Model file for the job. Use its own axes, mm. A direction names the side the tool comes from. Coordinates: 2 decimals unless noted, no trailing zeros. Loops run counter-clockwise (first coordinate to the right, second up) from the corner with the lowest first, then second, coordinate; pieces in that order, holes last. Notation, with made-up numbers: (38, 13) -> (92, 13) arc R16 ccw to (92, 29) -> close; hole circle Ø3 at (27, 34.5). An arc over 180 degrees is marked (long way). Use one line per item in the form item = value.
```python
from build123d import *

# Parameters (mm, degrees)
F0_W     = 38
F0_H     = 38
F1_DEPTH = 1.5
F2_R     = 2.25
F2_W     = 2.816632
F2_H     = 26.474444
F2_W_2   = 3.106516
F2_H_2   = 26.623748
F2_W_3   = 2.935091
F2_H_3   = 26.58009
F2_W_4   = 2.913202
F2_H_4   = 26.536286
F3_DEPTH = 1.501
F4_R     = 3
F5_R     = 1


with BuildPart() as f1:
    # F0 (on Top) → F1 (new body)
    with BuildSketch(Plane.XY):
        with Locations((-24.108174, 19)):
            Rectangle(F0_W, F0_H)
    extrude(amount=F1_DEPTH)

    # F2 (on face) → F3 (cut, through all)
    with BuildSketch(Plane.XY.offset(1.5)):
        with Locations((-39.408174, 34.3)):
            Circle(F2_R)
        with Locations((-8.808174, 34.3)):
            Circle(F2_R)
        with Locations((-8.808174, 3.7)):
            Circle(F2_R)
        with Locations((-39.408174, 3.7)):
            Circle(F2_R)
        with Locations((-34.555089, 19.259251)):
            Rectangle(F2_W, F2_H)
        with Locations((-27.583793, 19.268872)):
            Rectangle(F2_W_2, F2_H_2)
        with Locations((-19.434359, 19.247043)):
            Rectangle(F2_W_3, F2_H_3)
        with Locations((-12.618669, 19.225141)):
            Rectangle(F2_W_4, F2_H_4)
    extrude(amount=-F3_DEPTH, mode=Mode.SUBTRACT)

    # F4
    f4_edges = [f1.edges().sort_by_distance(p)[0] for p in [
        (-43.108174, 38, 0.75),
        (-5.108174, 38, 0.75),
        (-5.108174, 0, 0.75),
        (-43.108174, 0, 0.75),
    ]]
    fillet(f4_edges, radius=F4_R)

    # F5
    f5_edges = [f1.edges().sort_by_distance(p)[0] for p in [
        (-35.963405, 32.496473, 0.75),
        (-35.963405, 6.022029, 0.75),
        (-29.137051, 5.956998, 0.75),
        (-20.901905, 5.956998, 0.75),
        (-14.07527, 5.956998, 0.75),
        (-11.162068, 5.956998, 0.75),
        (-17.966814, 5.956998, 0.75),
        (-26.030535, 5.956998, 0.75),
        (-33.146773, 6.022029, 0.75),
        (-11.162068, 32.493284, 0.75),
        (-17.966814, 32.537088, 0.75),
        (-26.030535, 32.580746, 0.75),
        (-33.146773, 32.496473, 0.75),
        (-29.137051, 32.580746, 0.75),
        (-20.901905, 32.537088, 0.75),
        (-14.07527, 32.493284, 0.75),
    ]]
    fillet(f5_edges, radius=F5_R)


solid = f1.part
```
Q1. Which spindle directions (+Z, -Z, +X, -X, +Y, -Y) get a long thin tool onto all of the face, cutting with end or side? Do faces 4 (the face through (-27.6, 5.957, 0.8)), 5 (the face through (-24, 38, 1)). Say none if no direction does.
Result:
face_4 = +Z, -Z
face_5 = +Z, -Z, +X, -X, +Y
Q2. Wall check: line 1 along X through (y, z) = (28, 1.4); line 2 along X through (y, z) = (34.5, 0.4); line 3 along Y through (x, z) = (-12.5, 1). Give the ranges that are in metal, low to high.
Result:
line_1 = -43.11 to -35.96, -33.15 to -29.14, -26.03 to -20.9, -17.97 to -14.08, -11.16 to -5.11
line_2 = -43.11 to -41.65, -37.17 to -11.05, -6.57 to -5.11
line_3 = 0 to 5.96, 32.49 to 38
Q3. Mould opens along Y. For faces 1 (the face through (-28.836, 32.296, 0.74)), 2 (the face through (-42.25, 0.9, 0.76)), 3 (the face through (-43.108, 19, 1)) say: released by +Y, released by -Y, zero draft, split by the parting line, or undercut.
Result:
face_1 = undercut
face_2 = released by -Y
face_3 = zero draft
Q4. Band-saw the part on A-A, the plane y = 34.3. Write the cut outline in (x, z), and give its area (3 significant figures).
Result:
outline = (-43.11, 0) -> (-41.66, 0) -> (-41.66, 1.5) -> (-43.11, 1.5) -> close; (-37.16, 0) -> (-11.06, 0) -> (-11.06, 1.5) -> (-37.16, 1.5) -> close; (-6.56, 0) -> (-5.11, 0) -> (-5.11, 1.5) -> (-6.56, 1.5) -> close
area = 43.5 mm2
Q5. Pin check, flat tips, straight feed: pin 1 Ø7 at (x, y) = (-8.81, 3.7) entering from -Z; pin 2 Ø3.5 at (x, y) = (-8.81, 34.3) entering from -Z. Stop position of each tip, or through.
Result:
pin_1 = 0
pin_2 = through
Q6. Band-saw the part on C-C, the plane x = -35.5. Write the cut outline in (y, z), and give its area (3 significant figures).
Result:
outline = (0, 0) -> (6.18, 0) -> (6.18, 1.5) -> (0, 1.5) -> close; (32.34, 0) -> (38, 0) -> (38, 1.5) -> (32.34, 1.5) -> close
area = 17.8 mm2
Q7. Band-saw the part on B-B, the plane y = 18.5. Write the cut outline in (x, z).
Result:
outline = (-43.11, 0) -> (-35.96, 0) -> (-35.96, 1.5) -> (-43.11, 1.5) -> close; (-33.15, 0) -> (-29.14, 0) -> (-29.14, 1.5) -> (-33.15, 1.5) -> close; (-26.03, 0) -> (-20.9, 0) -> (-20.9, 1.5) -> (-26.03, 1.5) -> close; (-17.97, 0) -> (-14.08, 0) -> (-14.08, 1.5) -> (-17.97, 1.5) -> close; (-11.16, 0) -> (-5.11, 0) -> (-5.11, 1.5) -> (-11.16, 1.5) -> close
Q8. Band-saw the part on D-D, the plane z = 0.9. State how many separate pieces and enclosed holes the cut face has, and give its area (3 significant figures).
Result:
separate_pieces = 1
enclosed_holes = 8
area = 1,060 mm2
